The model under review builds one solid part; all positions refer to its coordinate system, in mm. A direction names the side the tool comes from. Round coordinates to 2 decimals unless told otherwise and drop trailing zeros. Write each loop counter-clockwise with the first axis right and the second up, starting at its lowest first coordinate (ties: lowest second). Pieces come first, ordered by that corner, then holes. Notation, with made-up numbers: M 10.5,24 L 19.5,24 A26 cw 19.5,44 Z; hole C 3.25,31 d10. An arc over 180 degrees is marked long. Write item = value, one per line. Start each with the question number.
Item 1: Take a section at A-A, the plane z = 0. Give the boundary of the cut face in (x, y), plus the area to 3 significant figures.
Item 2: To check wall thickness, follow line 1 along X through (y, z) = (5.5, 0.5); line 2 along Y through (x, z) = (-15, 49.5); line 3 along Y through (x, z) = (38.5, 3). State the ranges of each line that lie inside material, in increasing order.
Item 3: For pin 1 Ø6.5 at (x, z) = (-21.63, 66.57) entering from -Y; pin 2 Ø1.5 at (x, z) = (1.5, 19) entering from +Y; pin 3 Ø2 at (x, y) = (61.5, 2) entering from -Z; pin 4 Ø8 at (x, y) = (0.5, -7.5) entering from +Z, all flat-tipped, find the tip position at first contact; note any pin that passes through.
Item 4: The part is to be moulded in two halves that separate along X. For faces 1 (the flat face through (108, 0, 0)), 2 (the flat face through (-13, -16, 39)), 3 (the cylindrical face through (-23.477, -16.986, 63.025)), say which applies: +X half, -X half, draft (parallel to the pull), parting line (faces both ways), or undercut.
Item 5: Take a section at D-D, the plane x = 0. Give the boundary of the cut face in (y, z), plus the area to 3 significant figures.
Item 6: Take a section at B-B, the plane y = 0. Give the boundary of the cut face in (x, z) (3 decimals).
Item 7: Tool access review of faces 4 (the flat face through (-2, -20, -4)), 5 (the cylindrical face through (-3.905, 30.14, -0.867)), 6 (the cylindrical face through (56, 0, -5)): name each direction out of +Z, -Z, +X, -X, +Y, -Y from which nothing blocks a thin tool from reaching the whole face with its end or side.
Item 8: Take a section at C-C, the plane x = 99.5. Give the boundary of the cut face in (y, z).
from build123d import *

# Parameters (mm, degrees)
SKETCH1_R           = 4
BOSS_EXTRUDE1_DEPTH = 40
SKETCH3_R           = 8
BOSS_EXTRUDE2_DEPTH = 20
SKETCH4_R           = 5
BOSS_EXTRUDE3_DEPTH = 108
SKETCH5_W           = 14
SKETCH5_H           = 2
BOSS_EXTRUDE4_DEPTH = 80
CUT_EXTRUDE1_REACH  = 146.647
SKETCH6_R           = 4


with BuildPart() as part:
    # Sketch1 → Boss-Extrude1 (new, symmetric)
    with BuildSketch(Plane(origin=(0, 0, 0), x_dir=(1, 0, 0), z_dir=(0, 1, 0))):
        with Locations(Location((0, 0, 0), (0, 0, 270))):
            Circle(SKETCH1_R)
    extrude(amount=BOSS_EXTRUDE1_DEPTH, both=True)

    # Sketch3 → Boss-Extrude2 (add, symmetric)
    with BuildSketch(Plane(origin=(0, 0, 0), x_dir=(1, 0, 0), z_dir=(0, 1, 0))):
        with Locations(Location((0, 0, 0), (0, 0, 270))):
            Circle(SKETCH3_R)
    extrude(amount=BOSS_EXTRUDE2_DEPTH, both=True)

    # Sketch4 → Boss-Extrude3 (add)
    with BuildSketch(Plane(origin=(0, 0, 0), x_dir=(0, 0, -1), z_dir=(1, 0, 0))):
        with Locations(Location((0, 0, 0), (0, 0, 180))):
            Circle(SKETCH4_R)
    extrude(amount=BOSS_EXTRUDE3_DEPTH)

    # Sketch5 → Boss-Extrude4 (add)
    with BuildSketch(Plane(origin=(0, 0, 0), x_dir=(0.9510565162951534, 0, 0.3090169943749482), z_dir=(-0.3090169943749482, 0, 0.9510565162951534))):
        with Locations((0, -17)):
            Rectangle(SKETCH5_W, SKETCH5_H)
    extrude(amount=BOSS_EXTRUDE4_DEPTH)

    # Sketch6 → Cut-Extrude1 (cut, up to next)
    with BuildSketch(Plane(origin=(0, -16, 0), x_dir=(1, 0, 0), z_dir=(0, 1, 0)), mode=Mode.PRIVATE) as cut_extrude1_sk1:
        with Locations(Location((-21.631189606, -66.573956141, 0), (0, 0, 180))):
            Circle(SKETCH6_R)
    cut_extrude1_tool1 = extrude(cut_extrude1_sk1.sketch, amount=-CUT_EXTRUDE1_REACH, mode=Mode.PRIVATE) & part.part
    add(cut_extrude1_tool1.solids().sort_by_distance((-21.63119, -16, 66.573956))[0], mode=Mode.SUBTRACT)


solid = part.part
Response values:
q1.outline = M -8,-20 L -4,-20 L -4,-40 L 4,-40 L 4,-20 L 8,-20 L 8,-5 L 108,-5 L 108,5 L 8,5 L 8,20 L 4,20 L 4,40 L -4,40 L -4,20 L -8,20 Z
q1.area = 1,960 mm2
q2.line_1 = -7.98 to 7.98
q2.line_2 = -18 to -16
q2.line_3 = -4 to 4
q3.pin_1 = through
q3.pin_2 = -16
q3.pin_3 = -4.9
q3.pin_4 = 8
q4.face_1 = +X half
q4.face_2 = draft
q4.face_3 = undercut
q5.outline = M -40,-4 L -20,-4 L -20,-8 L 20,-8 L 20,-4 L 40,-4 L 40,4 L 20,4 L 20,8 L -16,8 L -16,22.65 L -18,22.65 L -18,8 L -20,8 L -20,4 L -40,4 Z
q5.area = 989 mm2
q6.outline = M 6.245,-5 L 108,-5 L 108,5 L 6.245,5 A8 ccw long Z
q7.face_4 = -Y
q7.face_5 = +Y
q7.face_6 = +X
q8.outline = C 0,0 d10
